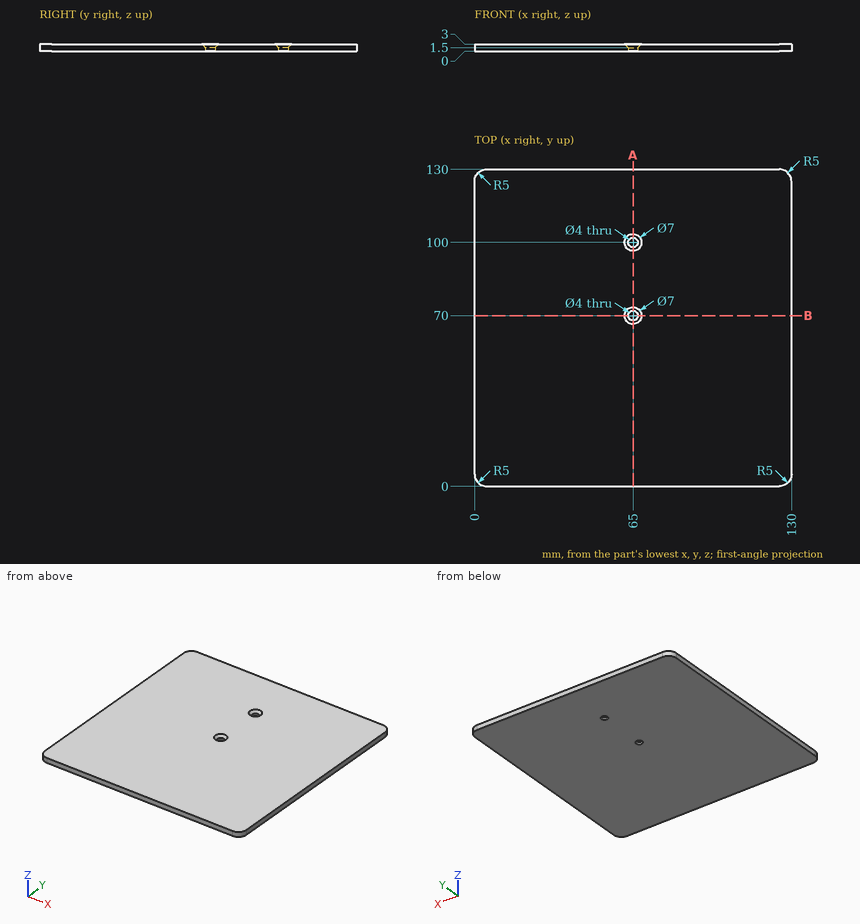
Print and shaded views of the part. All mm, measured from the part's lowest x, y and z. Round coordinates to 2 decimals unless told otherwise and drop trailing zeros. Write each loop counter-clockwise with the first axis right and the second up, starting at its lowest first coordinate (ties: lowest second). Pieces come first, ordered by that corner, then holes. Notation, with made-up numbers: M 14.5,-29 L 67.5,-29 A8 cw 67.5,-14 Z; hole C 1,15.5 d8. An arc over 180 degrees is marked long. One line per question, with ' | ' between items.
(1) Probe line 1 along Y through (x, z) = (65, 0.55); line 2 along X through (y, z) = (70, 1.05). List the from-to ranges inside material, lowest first.
Answer key:
line 1: y = 0 to 68, 72 to 98, 102 to 130 | line 2: x = 0 to 63, 67 to 130
(2) Saw through at A-A on x = 65. Write the cut outline in (y, z).
Answer key:
outline: M 0,0 L 68,0 L 68,1.5 L 66.5,3 L 0,3 Z; M 72,0 L 98,0 L 98,1.5 L 96.5,3 L 73.5,3 L 72,1.5 Z; M 102,0 L 130,0 L 130,3 L 103.5,3 L 102,1.5 Z
(3) Pin check, flat tip, straight feed: pin 1 (6.5 mm diameter, centred on x = 65, y = 100, fed in from +Z). Stop position of the tip, or through.
Answer key:
pin 1: stops at z = 2.75
(4) Saw through at B-B on y = 70. Write the cut outline in (x, z).
Answer key:
outline: M 0,0 L 63,0 L 63,1.5 L 61.5,3 L 0,3 Z; M 67,0 L 130,0 L 130,3 L 68.5,3 L 67,1.5 Z
